Here's how the part is built. I have some questions about the finished solid (model axes, mm). Coordinates: 2 decimals unless noted, no trailing zeros. Loops run counter-clockwise (first coordinate to the right, second up) from the corner with the lowest first, then second, coordinate; pieces in that order, holes last. Notation, with made-up numbers: (66.25, 14) -> (70.25, 14) arc R26 ccw to (70.25, 49) -> close; hole circle Ø4 at (-36.75, -26). An arc over 180 degrees is marked (long way). Answer as a JSON object with one key per item and string values. Group by question number.
Q1. I need wall thicknesses on line 1 (Y direction, x = -24, z = 2.75) (3 decimals); line 2 (X direction, y = 9, z = 1.25); line 3 (X direction, y = 8.5, z = 2.75). Which ranges of each line are inside material? Lowest first, please.
Q2. Thinking about a two-plate mould opening in X: for faces 1 (the conical face through (-0.11, -13.5, 6.46)), 2 (the conical face through (-37.313, 0.407, 0.319)), 3 (the flat face through (-8.4, 7.8, 7)), which applies, released by +X, released by -X, zero draft, split by the parting line, or undercut?
Q3. I'm going to push flat-ended pins straight in: pin 1 (4 mm diameter, centred on y = 2, z = 5.5, fed in from +X); pin 2 (4 mm diameter, centred on y = 11, z = 5.5, fed in from -X). Where does each tip first touch, or does it pass through?
Q4. I want a section at B-B on z = 4. Count the separate pieces of the cut face and the enclosed holes in it, then the cut area to 3 significant figures.
Q5. I want a section at A-A on x = -24. Write out the boundary of the cut face in (y, z) (3 decimals).
```python
from build123d import *

# Parameters (mm, degrees)
F1_DEPTH = 7
F2_R     = 6
F3_SIZE  = 2


# Not quite as in the source:
# - a feature names something its author has since deleted; it is built from what else it names


with BuildPart() as f1:
    # F0 (on Top) → F1 (new body)
    with BuildSketch(Plane.XY):
        with BuildLine():
            ThreePointArc((-14.0623969756, 5.1112299037), (-13.1615738007, 7.1167868393), (-11.9765766631, 8.9686839202))
            ThreePointArc((-11.9765766631, 8.9686839202), (-39, 0), (-11.9765766631, -8.9686839202))
            ThreePointArc((-11.9765766631, -8.9686839202), (-13.1615738007, -7.1167868393), (-14.0623969756, -5.1112299037))
            ThreePointArc((-14.0623969756, -5.1112299037), (-35.175, 0), (-14.0623969756, 5.1112299037))
        make_face()
        with BuildLine():
            ThreePointArc((-9.9141796875, -5.1565168597), (-11.175, 0), (-9.9141796875, 5.1565168597))
            ThreePointArc((-9.9141796875, 5.1565168597), (-10.8069599633, 7.1374851726), (-11.9765766631, 8.9686839202))
            ThreePointArc((-11.9765766631, 8.9686839202), (-13.1615738007, 7.1167868393), (-14.0623969756, 5.1112299037))
            ThreePointArc((-14.0623969756, 5.1112299037), (-13.1387537824, 2.6294401687), (-12.825, 0))
            ThreePointArc((-12.825, 0), (-13.1387537824, -2.6294401687), (-14.0623969756, -5.1112299037))
            ThreePointArc((-14.0623969756, -5.1112299037), (-13.1615738007, -7.1167868393), (-11.9765766631, -8.9686839202))
            ThreePointArc((-11.9765766631, -8.9686839202), (-10.8069599633, -7.1374851726), (-9.9141796875, -5.1565168597))
        make_face()
        with BuildLine():
            ThreePointArc((-9.9141796875, 5.1565168597), (0, 11.175), (9.9141796875, 5.1565168597))
            ThreePointArc((9.9141796875, 5.1565168597), (10.8069599633, 7.1374851726), (11.9765766631, 8.9686839202))
            ThreePointArc((11.9765766631, 8.9686839202), (0, 14.9624757252), (-11.9765766631, 8.9686839202))
            ThreePointArc((-11.9765766631, 8.9686839202), (-10.8069599633, 7.1374851726), (-9.9141796875, 5.1565168597))
        make_face()
        with BuildLine():
            ThreePointArc((9.9141796875, 5.1565168597), (10.8552195512, 2.6542105222), (11.175, 0))
            ThreePointArc((11.175, 0), (10.8552195512, -2.6542105222), (9.9141796875, -5.1565168597))
            ThreePointArc((9.9141796875, -5.1565168597), (10.8069599633, -7.1374851726), (11.9765766631, -8.9686839202))
            ThreePointArc((11.9765766631, -8.9686839202), (13.1615738007, -7.1167868393), (14.0623969756, -5.1112299037))
            ThreePointArc((14.0623969756, -5.1112299037), (12.825, 0), (14.0623969756, 5.1112299037))
            ThreePointArc((14.0623969756, 5.1112299037), (13.1615738007, 7.1167868393), (11.9765766631, 8.9686839202))
            ThreePointArc((11.9765766631, 8.9686839202), (10.8069599633, 7.1374851726), (9.9141796875, 5.1565168597))
        make_face()
        with BuildLine():
            ThreePointArc((39, 0), (28.724862429, 14.2364207239), (11.9765766631, 8.9686839202))
            ThreePointArc((11.9765766631, 8.9686839202), (13.1615738007, 7.1167868393), (14.0623969756, 5.1112299037))
            ThreePointArc((14.0623969756, 5.1112299037), (26.6294401687, 10.8612462176), (35.175, 0))
            ThreePointArc((35.175, 0), (26.6294401687, -10.8612462176), (14.0623969756, -5.1112299037))
            ThreePointArc((14.0623969756, -5.1112299037), (13.1615738007, -7.1167868393), (11.9765766631, -8.9686839202))
            ThreePointArc((11.9765766631, -8.9686839202), (28.724862429, -14.2364207239), (39, 0))
        make_face()
        with BuildLine():
            ThreePointArc((11.9765766631, -8.9686839202), (10.8069599633, -7.1374851726), (9.9141796875, -5.1565168597))
            ThreePointArc((9.9141796875, -5.1565168597), (0, -11.175), (-9.9141796875, -5.1565168597))
            ThreePointArc((-9.9141796875, -5.1565168597), (-10.8069599633, -7.1374851726), (-11.9765766631, -8.9686839202))
            ThreePointArc((-11.9765766631, -8.9686839202), (0, -14.9624757252), (11.9765766631, -8.9686839202))
        make_face()
    extrude(amount=F1_DEPTH)

    # F2
    f2_edges = [f1.edges().sort_by_distance(p)[0] for p in [
        (-11.976577, -8.968684, 3.5),
        (11.976577, -8.968684, 3.5),
        (11.976577, 8.968684, 3.5),
        (-11.976577, 8.968684, 3.5),
    ]]
    fillet(f2_edges, radius=F2_R)

    # F3
    f3_edges = [f1.edges().sort_by_distance(p)[0] for p in [
        (-39, 0, 0),
        (-39, 0, 7),
    ]]
    chamfer(f3_edges, length=F3_SIZE)


solid = f1.part
```
Result set:
{
 "1": {"line 1": "y = -15 to -11.175, 11.175 to 15", "line 2": "x = -35.05 to -30.62, -17.38 to -6.62, 6.62 to 17.38, 30.62 to 35.05", "line 3": "x = -36.36 to -31.25, -16.75 to -7.25, 7.25 to 16.75, 31.25 to 36.36"},
 "2": {"face 1": "undercut", "face 2": "undercut", "face 3": "zero draft"},
 "3": {"pin 1": "stops at x = 39", "pin 2": "stops at x = -35.95"},
 "4": {"separate pieces": "1", "enclosed holes": "3", "area": "815 mm²"},
 "5": {"outline": "(-15, 2) -> (-13, 0) -> (-11.175, 0) -> (-11.175, 7) -> (-13, 7) -> (-15, 5) -> close; (11.175, 0) -> (13, 0) -> (15, 2) -> (15, 5) -> (13, 7) -> (11.175, 7) -> close"}
}
